```python
from build123d import *

# Parameters (mm, degrees)
SKETCH_1_W          = 20
SKETCH_1_H          = 12
EXTRUDE_1_DEPTH     = 2.5
SKETCH_2_R          = 2
SKETCH_2_R_2        = 3.5
CUT_EXTRUDE_1_DEPTH = 24.457408211
SKETCH_3_R          = 0.5
CUT_EXTRUDE_3_DEPTH = 24.457408211
CUT_EXTRUDE_START   = -1
SKETCH_3_4_R        = 1.05
SKETCH_3_4_R_2      = 0.5
CUT_EXTRUDE_6_DEPTH = 1.5
EXTRUDE_2_DEPTH     = 6
SKETCH_5_R          = 0.4
CUT_EXTRUDE_7_DEPTH = 2


with BuildPart() as part:
    # 草图1 → 凸台-拉伸1 (new body)
    with BuildSketch(Plane(origin=(0, 0, 0), x_dir=(1, 0, 0), z_dir=(0, 1, 0))):
        with Locations((10, 6)):
            Rectangle(SKETCH_1_W, SKETCH_1_H)
    extrude(amount=EXTRUDE_1_DEPTH)

    # 草图2 → 切除-拉伸1 (cut, through all)
    with BuildSketch(Plane(origin=(0, 2.5, 0), x_dir=(1, 0, 0), z_dir=(0, 1, 0))):
        with Locations(Location((15, 6, 0), (0, 0, 270))):
            Circle(SKETCH_2_R)
        with Locations(Location((5, 6, 0), (0, 0, 270))):
            Circle(SKETCH_2_R_2)
    extrude(amount=-CUT_EXTRUDE_1_DEPTH, mode=Mode.SUBTRACT)

    # 草图3 → 切除-拉伸3 (cut, through all)
    with BuildSketch(Plane.XZ):
        with Locations(Location((18, -2, 0), (0, 0, 270))):
            Circle(SKETCH_3_R)
        with Locations(Location((18, -10, 0), (0, 0, 270))):
            Circle(SKETCH_3_R)
        with Locations(Location((10, -6, 0), (0, 0, 270))):
            Circle(SKETCH_3_R)
        with Locations(Location((5, -1.5, 0), (0, 0, 270))):
            Circle(SKETCH_3_R)
        with Locations(Location((5, -10.5, 0), (0, 0, 270))):
            Circle(SKETCH_3_R)
    extrude(amount=-CUT_EXTRUDE_3_DEPTH, mode=Mode.SUBTRACT)

    # 草图3<4> → 切除-拉伸6 (cut)
    # profile 1 of 5: a face of its own
    with BuildSketch(Plane.XZ.offset(CUT_EXTRUDE_START)):
        with Locations((5, -10.5)):
            Circle(SKETCH_3_4_R)
        with Locations(Location((5, -10.5, 0), (0, 0, 270))):
            Circle(SKETCH_3_4_R_2, mode=Mode.SUBTRACT)
    # profile 2 of 5: a face of its own
    with BuildSketch(Plane.XZ.offset(CUT_EXTRUDE_START)):
        with Locations((5, -1.5)):
            Circle(SKETCH_3_4_R)
        with Locations(Location((5, -1.5, 0), (0, 0, 270))):
            Circle(SKETCH_3_4_R_2, mode=Mode.SUBTRACT)
    # profile 3 of 5: a face of its own
    with BuildSketch(Plane.XZ.offset(CUT_EXTRUDE_START)):
        with Locations(Location((18, -2, 0), (0, 0, 90))):
            Circle(SKETCH_3_4_R)
        with Locations(Location((18, -2, 0), (0, 0, 270))):
            Circle(SKETCH_3_4_R_2, mode=Mode.SUBTRACT)
    # profile 4 of 5: a face of its own
    with BuildSketch(Plane.XZ.offset(CUT_EXTRUDE_START)):
        with Locations(Location((10, -6, 0), (0, 0, 90))):
            Circle(SKETCH_3_4_R)
        with Locations(Location((10, -6, 0), (0, 0, 270))):
            Circle(SKETCH_3_4_R_2, mode=Mode.SUBTRACT)
    # profile 5 of 5: a face of its own
    with BuildSketch(Plane.XZ.offset(CUT_EXTRUDE_START)):
        with Locations(Location((18, -10, 0), (0, 0, 90))):
            Circle(SKETCH_3_4_R)
        with Locations(Location((18, -10, 0), (0, 0, 270))):
            Circle(SKETCH_3_4_R_2, mode=Mode.SUBTRACT)
    extrude(amount=-CUT_EXTRUDE_6_DEPTH, mode=Mode.SUBTRACT)

    # 草图4 → 凸台-拉伸2 (add)
    with BuildSketch(Plane(origin=(0, 2.5, 0), x_dir=(1, 0, 0), z_dir=(0, 1, 0))):
        with BuildLine():
            Line((15, 11.75), (15, 12))
            Line((15, 12), (5, 12))
            Line((5, 12), (5, 11.75))
            ThreePointArc((5, 11.75), (7.892718316, 10.969374281), (10, 8.839454173))
            ThreePointArc((10, 8.839454173), (12.107281684, 10.969374281), (15, 11.75))
        make_face()
        with BuildLine():
            Line((15, 0), (15, 0.25))
            ThreePointArc((15, 0.25), (12.107281684, 1.030625719), (10, 3.160545827))
            ThreePointArc((10, 3.160545827), (7.892718316, 1.030625719), (5, 0.25))
            Line((5, 0.25), (5, 0))
            Line((5, 0), (15, 0))
        make_face()
    extrude(amount=EXTRUDE_2_DEPTH)

    # 草图5 → 切除-拉伸7 (cut)
    with BuildSketch(Plane(origin=(0, 8.5, 0), x_dir=(1, 0, 0), z_dir=(0, 1, 0))):
        with Locations(Location((10, 1.2, 0), (0, 0, 270))):
            Circle(SKETCH_5_R)
        with Locations(Location((10, 10.8, 0), (0, 0, 270))):
            Circle(SKETCH_5_R)
    extrude(amount=-CUT_EXTRUDE_7_DEPTH, mode=Mode.SUBTRACT)


solid = part.part
```
Source: CAD feature listing. Evaluate the final solid. Frame: model axes, mm. A direction names the side the tool comes from. Round coordinates to 2 decimals unless told otherwise and drop trailing zeros. Write each loop counter-clockwise with the first axis right and the second up, starting at its lowest first coordinate (ties: lowest second). Pieces come first, ordered by that corner, then holes. Notation, with made-up numbers: M 6,-39.5 L 12,-39.5 A31 ccw 12,-13.5 Z; hole C 48,40.5 d5. An arc over 180 degrees is marked long. Answer as a JSON object with one key per item and string values. Group by question number.
(1) Section query C-C on y = 4. Output: boundary loops of the cut face in (x, z), then the cut area to 3 significant figures.
(2) Reachability of faces 1 (the flat face through (10, 8.5, -0.5)), 2 (the cylindrical face through (7.86, 5.46, -10.99)), 3 (the cylindrical face through (9.85, 7.51, -10.43)), 4 (the cylindrical face through (12.14, 5.46, -1.01)) from +Z, -Z, +X, -X, +Y, -Y: full face, straight path, thin tool, end or side. Return the list, or none.
(3) Section query D-D on z = -1.25. Output: boundary loops of the cut face in (x, y).
(4) Section query B-B on x = 18. Output: boundary loops of the cut face in (y, z).
(5) First-contact query: pin 1 (1.3 mm diameter, centred on x = 5, z = -1.5, fed in from +Y); pin 2 (1.3 mm diameter, centred on x = 5, z = -10.5, fed in from -Y); pin 3 (2.5 mm diameter, centred on x = 10, z = -6, fed in from +Y); pin 4 (2 mm diameter, centred on y = 7, z = -8, fed in from -X). Flat tips, straight axial feed; report the tip coordinate or a pass-through.
(6) Mould query, pull axis Z, two halves, no side actions, for faces 5 (the flat face through (10, 3, 0)), 6 (the flat face through (0, 1, -6)), 7 (the cylindrical face through (5.496, 0.493, -1.435)), 8 (the flat face through (10, 3, -12)). Classes: +Z half, -Z half, draft (parallel to the pull), parting line (faces both ways), or undercut.
(7) Section query A-A on y = 7.5. Output: boundary loops of the cut face in (x, z).
(8) Ray query, line 1 (X direction, y = 1.7, z = -6); line 2 (Z direction, x = 18, y = 1.7); line 3 (X direction, y = 1.4, z = -2). Return the intervals inside material, ascending. Write a range as [from, to].
Computed values:
{
 "1": {"outline": "M 5,-12 L 15,-12 L 15,-11.75 A5.75 cw 10,-8.84 A5.75 cw 5,-11.75 Z; M 5,-0.25 A5.75 cw 10,-3.16 A5.75 cw 15,-0.25 L 15,0 L 5,0 Z", "area": "21.9 mm^2"},
 "2": {"face 1": "+Z, -Z, +X, -X, +Y", "face 2": "-X, +Y", "face 3": "+Y", "face 4": "+X, +Y"},
 "3": {"outline": "M 0,0 L 4.57,0 L 4.57,1 L 3.98,1 L 3.98,2.5 L 0,2.5 Z; M 5.43,0 L 20,0 L 20,2.5 L 18.73,2.5 L 18.73,1 L 17.27,1 L 17.27,2.5 L 11.76,2.5 L 11.76,8.5 L 10.4,8.5 L 10.4,6.5 L 9.6,6.5 L 9.6,8.5 L 8.24,8.5 L 8.24,2.5 L 6.02,2.5 L 6.02,1 L 5.43,1 Z"},
 "4": {"outline": "M 0,-12 L 2.5,-12 L 2.5,-11.05 L 1,-11.05 L 1,-10.5 L 0,-10.5 Z; M 0,-9.5 L 1,-9.5 L 1,-8.95 L 2.5,-8.95 L 2.5,-3.05 L 1,-3.05 L 1,-2.5 L 0,-2.5 Z; M 0,-1.5 L 1,-1.5 L 1,-0.95 L 2.5,-0.95 L 2.5,0 L 0,0 Z"},
 "5": {"pin 1": "y = 1", "pin 2": "y = 0", "pin 3": "y = 2.5", "pin 4": "x = 9.91"},
 "6": {"face 5": "+Z half", "face 6": "draft", "face 7": "undercut", "face 8": "-Z half"},
 "7": {"outline": "M 5,-12 L 15,-12 L 15,-11.75 A5.75 cw 10,-8.84 A5.75 cw 5,-11.75 Z; M 5,-0.25 A5.75 cw 10,-3.16 A5.75 cw 15,-0.25 L 15,0 L 5,0 Z; hole C 10,-10.8 d0.8; hole C 10,-1.2 d0.8"},
 "8": {"line 1": "[0, 1.5], [8.5, 8.95], [11.05, 13], [17, 20]", "line 2": "[-12, -11.05], [-8.95, -3.05], [-0.95, 0]", "line 3": "[0, 4.08], [5.92, 16.95], [19.05, 20]"}
}
